Read the model definition and answer for the solid it produces. Units are mm, in the model's axes. Face numbers are marked on the shaded views. A direction names the side the tool comes from. Coordinates: 2 decimals unless noted, no trailing zeros. Order: outer loops, then holes, each group sorted by start corner. A loop starts at its lowest first (then second) coordinate and runs counter-clockwise, first axis right, second up. Notation, with made-up numbers: (69.25, 44) -> (77.25, 44) arc R10 cw to (77.25, 49) -> close; hole circle Ø9 at (-6, 53). An arc over 180 degrees is marked (long way). Return JSON: item names as keys, results as strings. Group by question number.
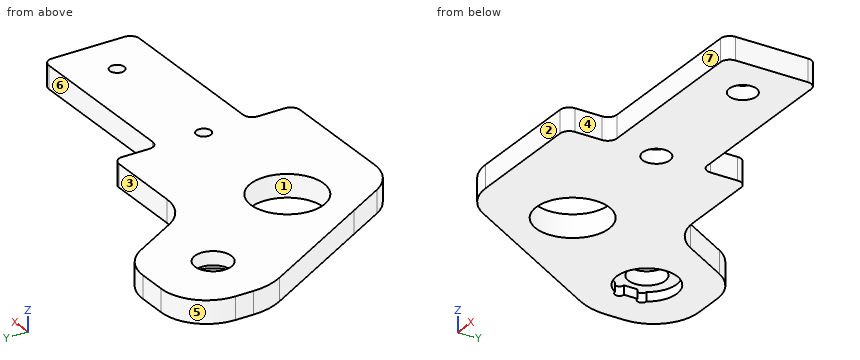
Autodesk Inventor part; units mm, degrees
ref_plane "YZ Plane" through (0, 0, 0) normal (1, 0, 0) x (0, 1, 0)
ref_plane "XZ Plane" through (0, 0, 0) normal (0, 1, 0) x (-1, 0, 0)
ref_plane "XY Plane" through (0, 0, 0) normal (0, 0, 1) x (1, 0, 0)
sketch "スケッチ1" plane through (0, 0, 0) normal (0, 0, 1) x (1, 0, 0)
  line L0 (0, 0) -> (98, 0)
  line L1 (98, 0) -> (98, 60)
  line L2 (98, 60) -> (0, 60)
  line L3 (0, 60) -> (0, 0)
  line L4 (98, 0) -> (29, 0)
  line L5 (29, 0) -> (29, 40)
  line L6 (29, 40) -> (98, 40)
  line L7 (98, 40) -> (98, 0)
  line L8 (29, 30) -> (98, 30)
  line L9 (98, 30) -> (98, 10)
  line L10 (98, 10) -> (29, 10)
  line L11 (29, 10) -> (29, 30)
  line L12 (98, 20) -> (0, 20)
  line L13 (29, 20) -> (5.906, 60)
  circle A0 centre (29, 20) radius 8.025
  circle A1 centre (14, 45.9808) radius 4.025
  line L14 (58, 40) -> (58, 0)
  line L15 (16.8756, 13) -> (-6.2184, 53)
  line L16 (41.1244, 27) -> (18.0303, 67)
  circle A2 centre (14, 45.9808) radius 14
  line L17 (16.8756, 13) -> (25.3526, -1.6825)
  point P0 (58, 30)
  point P1 (33.6188, 40)
  point P2 (22.0718, 60)
  point P3 (0, 45.9808)
  point P4 (1.8756, 38.9808)
  point P5 (24.3812, 0)
  point P6 (58, 0)
  point P7 (58, 10)
  dimension "d0" = 98
  dimension "d1" = 60
  dimension "d2" = 40
  dimension "d3" = 20
  dimension "d4" = 10
  dimension "d5" = 69
  dimension "d6" = 30
  dimension "d7" = 16.05
  dimension "d8" = 30
  dimension "d9" = 8.05
  dimension "d10" = 40
  dimension "d11" = 28
extrude "押し出し1" add sketch "スケッチ1" along normal blind 5 contours L5 L10 L14 L0 | L0 L17 L15 L12 A0 L5 | L5 A0 L12 L14 L10 | L14 L12 L1 L10 | L14 L8 L1 L12 | L12 A0 L5 L8 L14 | L15 A2 L13 A0 L12 | L8 L16 L6 L14 | A2 L13 A1 | A0 L13 A2 L16 L6 L5 | L8 L5 L6 L16 | L3 L2 L13 A2 | L13 A1 A2 | L13 L2 L16 A2
sketch "スケッチ2" plane through (0, 0, 5) normal (0, 0, 1) x (1, 0, 0)
  line L0 (98, 10) -> (98, 30)
  line L1 (98, 20) -> (47.1161, 20)
  point P0 (0, 0)
  point P1 (88, 20)
  point P2 (58, 20)
  dimension "d14" = 10
  dimension "d15" = 30
hole "穴1" at (88, 20, 5) at (58, 20, 5) direction (0, 0, -1) diameter 3.2 depth 10
fillet "フィレット1" radius 2 6 edges at (58, 40, 2.5) (58, 30, 2.5) (98, 30, 2.5) (98, 10, 2.5) (58, 0, 2.5) (58, 10, 2.5)
fillet "フィレット2" radius 10 4 edges at (24.3812, 0, 2.5) (0, 60, 2.5) (22.0718, 60, 2.5) (33.6188, 40, 2.5)
sketch "スケッチ5" plane through (0, 0, 0) normal (0, 0, -1) x (-1, 0, 0)
  circle A0 centre (-88, 20) radius 1.6
  circle A1 centre (-88, 20) radius 3
  circle A2 centre (-58, 20) radius 1.6
  circle A3 centre (-58, 20) radius 3
  point P0 (0, 0)
  dimension "d38" = 6
  dimension "d39" = 6
extrude "押し出し3" cut sketch "スケッチ5" against normal blind 3 contours A0 | A1 | A2 | A3
sketch "スケッチ6" plane through (0, 0, 0) normal (0, 0, -1) x (-1, 0, 0)
  circle A0 centre (-14, 45.9808) radius 4.025
  circle A1 centre (-14, 45.9808) radius 6.6
  line L0 (-8.4, 49.4736) -> (-8.4, 42.4879)
  arc A2 (-8.4, 47.4736) -> (-8.4, 49.4736) centre (-8.4, 48.4736) ccw
  arc A3 (-8.4, 42.4879) -> (-8.4, 44.4879) centre (-8.4, 43.4879) ccw
  point P0 (0, 0)
  dimension "d42" = 13.2
  dimension "d45" = 5.6
  dimension "d46" = 1
  dimension "d47" = 0
  dimension "d48" = 0
  dimension "d49" = 1
extrude "押し出し4" cut sketch "スケッチ6" against normal blind 2 contours L0 A1 | A2 A1 | A1 A2 L0 | L0 A3 A1 | A1 A3
equation "\"d49\" = d46"
properties part number "RP_Calf-Link-cover-Inside-Right"
1. For a pull along Y with two mould halves and no side action, classify the marked faces 1, 2, 3 and 4 as released by +Y, released by -Y, zero draft, split by the parting line, or undercut.
2. Straight lines are drawn through the part: L1, parallel to X at y = 22.5, z = 1.4; L2, parallel to Y at x = 15.5, z = 2.35; L3, parallel to Y at x = 14, z = 2.85. For each, find the intervals that lie inside material, in ascending order.
3. Find section B-B on z = 3.9. Determine the outline of the cut face in (x, y) (3 decimals), and give its area (3 significant figures).
4. Find section D-D on x = 65. Determine the outline of the cut face in (y, z), and give its area (3 significant figures).
5. Find section C-C on x = 29. Determine the outline of the cut face in (y, z) (3 decimals).
6. Given pin 1 (1.5 mm diameter, centred on x = 80.5, z = 2.5, fed in from +Y); pin 2 (1.8 mm diameter, centred on x = 58.5, y = 21.5, fed in from -Z); pin 3 (0.6 mm diameter, centred on y = 46, z = 1, fed in from +X), each flat-ended and moving along its own axis, determine where each tip first touches the part or whether it passes through.
7. Find section A-A on x = 88. Determine the outline of the cut face in (y, z), and give its area (3 significant figures).
8. Which of the six approach directions +Z, -Z, +X, -X, +Y, -Y give full straight-line access (tool end or side, diameter ignored) to the marked faces 5, 6 and 7?
Result:
{
 "1": {"face 1": "undercut", "face 2": "released by -Y", "face 3": "released by +Y", "face 4": "zero draft"},
 "2": {"L1": "11.39 to 21.37, 36.63 to 56.34, 59.66 to 86.34, 89.66 to 98", "L2": "15.38 to 42.25, 49.72 to 60", "L3": "17.98 to 41.96, 50.01 to 60"},
 "3": {"outline": "(0, 45.981) arc R14 ccw to (1.876, 38.981) -> (16.876, 13) -> (21.494, 5) arc R10 ccw to (30.155, 0) -> (56, 0) arc R2 ccw to (58, 2) -> (58, 8) arc R2 cw to (60, 10) -> (96, 10) arc R2 ccw to (98, 12) -> (98, 28) arc R2 ccw to (96, 30) -> (60, 30) arc R2 cw to (58, 32) -> (58, 38) arc R2 ccw to (56, 40) -> (39.392, 40) arc R10 cw to (30.732, 45) -> (24.959, 55) arc R10 ccw to (16.298, 60) -> (10, 60) arc R10 ccw to (0, 50) -> close; hole circle Ø8.05 at (14, 45.981); hole circle Ø16.05 at (29, 20); hole circle Ø3.2 at (58, 20); hole circle Ø3.2 at (88, 20)", "area": "2,860 mm^2"},
 "4": {"outline": "(10, 0) -> (30, 0) -> (30, 5) -> (10, 5) -> close", "area": "100 mm^2"},
 "5": {"outline": "(0.067, 0) -> (11.975, 0) -> (11.975, 5) -> (0.067, 5) -> close; (28.025, 0) -> (48, 0) -> (48, 5) -> (28.025, 5) -> close"},
 "6": {"pin 1": "y = 30", "pin 2": "z = 3", "pin 3": "x = 30.33"},
 "7": {"outline": "(10, 0) -> (17, 0) -> (17, 3) -> (18.4, 3) -> (18.4, 5) -> (10, 5) -> close; (21.6, 3) -> (23, 3) -> (23, 0) -> (30, 0) -> (30, 5) -> (21.6, 5) -> close", "area": "75.6 mm^2"},
 "8": {"face 5": "+Z, -Z, -X, +Y", "face 6": "+Z, -Z, +X, +Y", "face 7": "+Z, -Z, +X, -Y"}
}
